from build123d import *

# Parameters (mm, degrees)
BOSS_EXTRU_1_DEPTH      = 6.35
ESQUISSE3_W             = 12.7
ESQUISSE3_H             = 12.7
ENL_V_MAT_EXTRU_1_DEPTH = 198.361432403
ENL_V_MAT_EXTRU_2_DEPTH = 198.361432403
CONG_1_R                = 6.35


with BuildPart() as part:
    # Esquisse2 → Boss.-Extru.1 (new body)
    with BuildSketch(Plane.XY):
        Polygon((6.35, -190.5), (12.7, -190.5), (12.7, 190.5), (-12.7, 190.5), (-12.7, -190.5), (-6.35, -190.5), (-6.35, -196.85), (6.35, -196.85), align=None)
    extrude(amount=BOSS_EXTRU_1_DEPTH)

    # Esquisse3 → Enlèv. mat.-Extru.1 (cut, through all)
    with BuildSketch(Plane.XY.offset(6.35)):
        with Locations((0, -106.82478)):
            Rectangle(ESQUISSE3_W, ESQUISSE3_H)
    extrude(amount=-ENL_V_MAT_EXTRU_1_DEPTH, mode=Mode.SUBTRACT)

    # Esquisse4 → Enlèv. mat.-Extru.2 (cut, through all)
    with BuildSketch(Plane.XY.offset(6.35)):
        with BuildLine():
            Line((2.75, 165.1), (2.75, 38.1))
            ThreePointArc((2.75, 38.1), (0, 35.35), (-2.75, 38.1))
            Line((-2.75, 38.1), (-2.75, 165.1))
            ThreePointArc((-2.75, 165.1), (0, 167.85), (2.75, 165.1))
        make_face()
    extrude(amount=-ENL_V_MAT_EXTRU_2_DEPTH, mode=Mode.SUBTRACT)

    # Congé1
    cong_1_edges = [part.edges().sort_by_distance(p)[0] for p in [
        (-12.7, 190.5, 3.175),
        (12.7, 190.5, 3.175),
    ]]
    fillet(cong_1_edges, radius=CONG_1_R)


solid = part.part
The listing builds one solid part. Answer for the finished solid, in the listing's coordinates (mm). A direction names the side the tool comes from. Coordinates: 2 decimals unless noted, no trailing zeros. Loops run counter-clockwise (first coordinate to the right, second up) from the corner with the lowest first, then second, coordinate; pieces in that order, holes last. Notation, with made-up numbers: M 18,4 L 40,4 A22 cw 40,40 Z; hole C 85,35.25 d2. An arc over 180 degrees is marked long. Answer in a Markdown table with one row per item.
1) Given pin 1 (1.9 mm diameter, centred on x = -10.5, z = 2.5, fed in from -Y); pin 2 (1.5 mm diameter, centred on x = 9.5, z = 1, fed in from +Y), each flat-ended and moving along its own axis, determine where each tip first touches the part or whether it passes through.
Answers below:
| item | result |
|---|---|
| pin 1 | y = -190.5 |
| pin 2 | y = 190.03 |
2) Find the intervals of material crossed by probe 1 along Y at (x, z) = (5.25, 0.5); probe 2 along X at (y, z) = (161, 1.75); probe 3 along Y at (x, z) = (1.5, 5.25), in increasing order.
Answers below:
| item | result |
|---|---|
| probe 1 | -196.85 to -113.17, -100.47 to 190.5 |
| probe 2 | -12.7 to -2.75, 2.75 to 12.7 |
| probe 3 | -196.85 to -113.17, -100.47 to 35.8, 167.4 to 190.5 |
3) Which of the six approach directions +Z, -Z, +X, -X, +Y, -Y give full straight-line access (tool end or side, diameter ignored) to faces 1 (the flat face through (-2.75, 101, 3)), 2 (the flat face through (9, -190.5, 3)), 3 (the flat face through (-10, -190.5, 3))?
Answers below:
| item | result |
|---|---|
| face 1 | +Z, -Z |
| face 2 | +Z, -Z, +X, -Y |
| face 3 | +Z, -Z, -X, -Y |
4) Find section A-A (z = 2.75). Determine the outline of the cut face in (x, y).
Answers below:
| item | result |
|---|---|
| outline | M -12.7,-190.5 L -6.35,-190.5 L -6.35,-196.85 L 6.35,-196.85 L 6.35,-190.5 L 12.7,-190.5 L 12.7,184.15 A6.35 ccw 6.35,190.5 L -6.35,190.5 A6.35 ccw -12.7,184.15 Z; hole M -6.35,-113.17 L 6.35,-113.17 L 6.35,-100.47 L -6.35,-100.47 Z; hole M -2.75,38.1 A2.75 ccw 2.75,38.1 L 2.75,165.1 A2.75 ccw -2.75,165.1 Z |
5) Find section B-B (y = 141). Determine the outline of the cut face in (x, z).
Answers below:
| item | result |
|---|---|
| outline | M -12.7,0 L -2.75,0 L -2.75,6.35 L -12.7,6.35 Z; M 2.75,0 L 12.7,0 L 12.7,6.35 L 2.75,6.35 Z |
6) Determine the mould class of faces 4 (the flat face through (2.75, 102, 3)), 5 (the flat face through (0, 0, 0)), 6 (the flat face through (-6.35, -194, 3)), 7 (the cylindrical face through (10.89, 188.59, 3.22)) for opening direction X: released by +X, released by -X, zero draft, split by the parting line, or undercut.
Answers below:
| item | result |
|---|---|
| face 4 | undercut |
| face 5 | zero draft |
| face 6 | released by -X |
| face 7 | released by +X |
